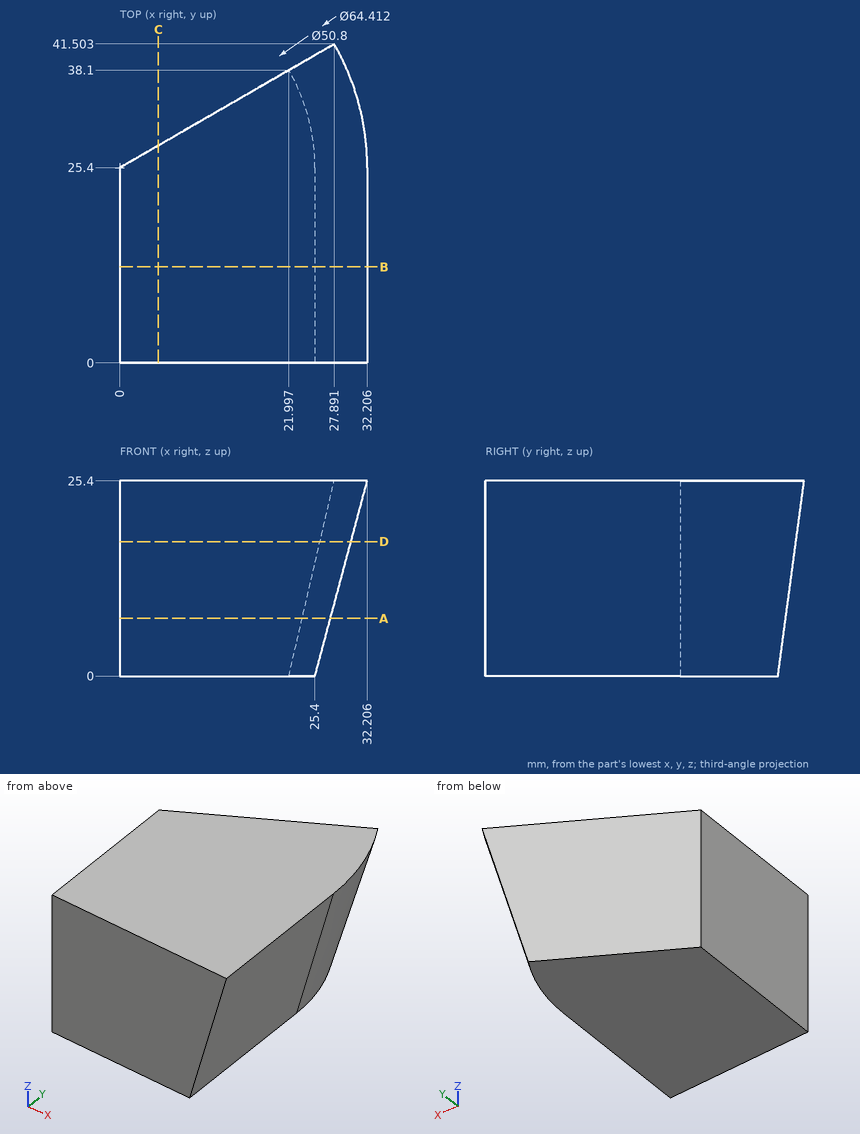
Source: three-view drawing plus pictorial views. Frame: mm from the lowest corner of the part. Round coordinates to 2 decimals unless told otherwise and drop trailing zeros. Write each loop counter-clockwise with the first axis right and the second up, starting at its lowest first coordinate (ties: lowest second). Pieces come first, ordered by that corner, then holes. Notation, with made-up numbers: M -37,-33 L -3,-33 A21 ccw -3,-24 Z; hole C 84,-16 d10. An arc over 180 degrees is marked long. Write each question's results on one line, items separated by ' | '.
Q1. Section query B-B (y = 12.5). Return loops of the section in (x, z), and give its area (3 significant figures).
Results:
outline: M 0,0 L 25.4,0 L 32.21,25.4 L 0,25.4 Z | area: 732 mm^2
Q2. Section query D-D (z = 17.5). Return loops of the section in (x, y), and give its area (3 significant figures).
Results:
outline: M 0,0 L 30.09,0 L 30.09,25.4 A30.09 ccw 26.06,40.44 L 0,25.4 Z | area: 1,000 mm^2
Q3. Section query A-A (z = 7.5). Return loops of the section in (x, y) (1 decimal).
Results:
outline: M 0,0 L 27.4,0 L 27.4,25.4 A27.4 ccw 23.7,39.1 L 0,25.4 Z
Q4. Section query C-C (x = 5). Return loops of the section in (y, z).
Results:
outline: M 0,0 L 28.29,0 L 28.29,25.4 L 0,25.4 Z
Q5. Pin query (flat end, axial travel): P1, Ø1, axis at y = 23.5, z = 5.5, coming from the +X side; P2, Ø2, axis at x = 15.5, z = 14, coming from the -Y side; P3, Ø4, axis at y = 29, z = 15, coming from the -X side; P4, Ø8, axis at y = 7.5, z = 4, coming from the +X side. Return the tip coordinate at first contact, or that it passes through.
Results:
P1: stops at x = 27.01 | P2: stops at y = 0 | P3: stops at x = 2.77 | P4: stops at x = 27.54
Q6. Line query: line 1 along X through (y, z) = (10, 16.25); line 2 along Y through (x, z) = (13, 1.75) (1 decimal); line 3 along X through (y, z) = (28, 4) (1 decimal). Output: solid intervals per line, ascending.
Results:
line 1: x = 0 to 29.75 | line 2: y = 0 to 32.9 | line 3: x = 4.5 to 26.3
